Geometry: see drawing. Coordinates: mm, zero at the bounding-box minimum. A direction names the side the tool comes from. Give positions to 0.01 mm unless a question says otherwise; leave off trailing zeros. Write each loop counter-clockwise with the first axis right and the second up, starting at its lowest first coordinate (ties: lowest second). Pieces come first, ordered by that corner, then holes. Notation, with made-up numbers: M 16,68 L 59,68 A28 cw 59,94 Z; hole C 38,14.5 d11. An arc over 180 degrees is marked long. Answer as a JSON object with one key per item and string values. Group by question number.
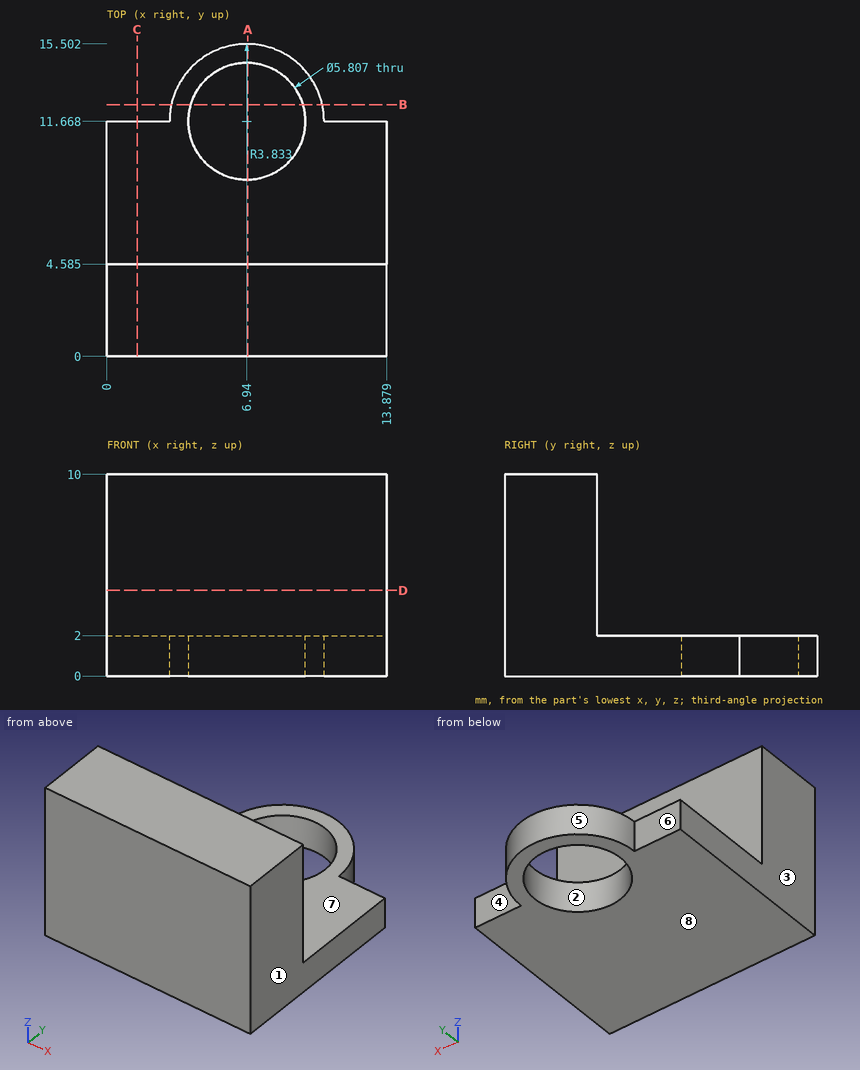
(1) Section C-C, the plane x = 1.5. Return loops of the section in (y, z) (1 decimal).
(2) Section D-D, the plane z = 4.25. Return loops of the section in (x, y) (1 decimal).
(3) Access query for the marked faces 4, 5, 6, 7 and 8. Directions: +Z, -Z, +X, -X, +Y, -Y. A direction counts if a zero-diameter tool reaches every point of the face in a straight line with its end or side. Return the directions, or none.
(4) Contact query for flat-ended pins moving along their axis: pin 1 Ø5.5 at (x, y) = (8.5, 11) entering from +Z; pin 2 Ø1.6 at (x, z) = (12, 1) entering from +Y; pin 3 Ø5 at (x, z) = (9, 7.5) entering from +Y (1 decimal). Output: stop coordinate, or through.
(5) Section B-B, the plane y = 12.5. Return loops of the section in (x, z).
(6) Section A-A, the plane x = 7. Return loops of the section in (y, z) (1 decimal).
(7) Pull-direction query (X, two-part tool) for the marked faces 1, 2 and 3; classes: pulls with the +X half, pulls with the -X half, needs draft (parallel to the pull), parting line crosses it, or undercut.
(8) Ray query, L1, parallel to Y at x = 4, z = 3.25 (1 decimal); L2, parallel to Z at x = 5.75, y = 8.5; L3, parallel to Y at x = 5.25, z = 1.5 (1 decimal). Return the intervals inside material, ascending. Write a range as [from, to].
Reported:
{
 "1": {"outline": "M 0,0 L 11.7,0 L 11.7,2 L 4.6,2 L 4.6,10 L 0,10 Z"},
 "2": {"outline": "M 0,0 L 13.9,0 L 13.9,4.6 L 0,4.6 Z"},
 "3": {"face 4": "+Z, -Z, +X, +Y", "face 5": "+Z, -Z, +Y", "face 6": "+Z, -Z, -X, +Y", "face 7": "+Z, +X, -X, +Y", "face 8": "-Z, +X, -X, +Y, -Y"},
 "4": {"pin 1": "stops at z = 2", "pin 2": "stops at y = 11.67", "pin 3": "stops at y = 4.6"},
 "5": {"outline": "M 3.2,0 L 4.16,0 L 4.16,2 L 3.2,2 Z; M 9.72,0 L 10.68,0 L 10.68,2 L 9.72,2 Z"},
 "6": {"outline": "M 0,0 L 8.8,0 L 8.8,2 L 4.6,2 L 4.6,10 L 0,10 Z; M 14.6,0 L 15.5,0 L 15.5,2 L 14.6,2 Z"},
 "7": {"face 1": "pulls with the +X half", "face 2": "undercut", "face 3": "pulls with the -X half"},
 "8": {"L1": "y = [0, 4.6]", "L2": "z = [0, 2]", "L3": "y = [0, 9.3], [14, 15.1]"}
}
